```python
from build123d import *

# Parameters (mm, degrees)
PAD_DEPTH       = 7
PAD012_DEPTH    = 25
SKETCH013_R     = 5
SKETCH013_R_2   = 3
POCKET007_DEPTH = 7.001
POCKET008_DEPTH = 30
SKETCH023_R     = 5
POCKET009_DEPTH = 4
SKETCH024_R     = 4.5
PAD013_DEPTH    = 30
SKETCH028_R     = 2.75
POCKET012_DEPTH = 1.5
SKETCH029_R     = 1.55
POCKET013_DEPTH = 32.001
SKETCH030_R     = 2.5
POCKET014_DEPTH = 3
POCKET015_DEPTH = 25.001


with BuildPart() as part:
    # Sketch011 → Pad (new body)
    with BuildSketch(Plane.XZ):
        with BuildLine():
            Line((73.255, 35.51), (73.255, 5))
            ThreePointArc((68.255, 0), (71.790534, 1.464466), (73.255, 5))
            Line((68.255, 0), (-68.255, 0))
            ThreePointArc((-73.255, 5), (-71.790534, 1.464466), (-68.255, 0))
            Line((-73.255, 5), (-73.255, 35.51))
            Line((-73.255, 35.51), (-81.66, 35.51))
            ThreePointArc((-86.66, 40.51), (-85.195534, 36.974466), (-81.66, 35.51))
            Line((-86.66, 40.51), (-86.66, 79.371844))
            ThreePointArc((-79.132903, 89.061258), (-84.557121, 85.50662), (-86.66, 79.371844))
            ThreePointArc((79.132903, 89.061258), (0, 99), (-79.132903, 89.061258))
            ThreePointArc((86.66, 79.371844), (84.557121, 85.50662), (79.132903, 89.061258))
            Line((86.66, 79.371844), (86.66, 40.51))
            ThreePointArc((81.66, 35.51), (85.195534, 36.974466), (86.66, 40.51))
            Line((81.66, 35.51), (73.255, 35.51))
        make_face()
    extrude(amount=PAD_DEPTH)

    # Sketch012 → Pad012 (join)
    with BuildSketch(Plane.XZ):
        with BuildLine():
            ThreePointArc((79.132903, 89.061258), (0, 99), (-79.132903, 89.061258))
            ThreePointArc((-79.132903, 89.061258), (-84.557121, 85.50662), (-86.66, 79.371844))
            Line((-86.66, 79.371844), (-86.66, 40.51))
            ThreePointArc((-86.66, 40.51), (-85.195534, 36.974466), (-81.66, 35.51))
            Line((-81.66, 35.51), (-73.255, 35.51))
            Line((-73.255, 35.51), (-73.255, 28.649016))
            ThreePointArc((-73.255, 28.649016), (-53.725584, 32.7828), (-34.688969, 38.790593))
            ThreePointArc((34.688969, 38.790593), (0, 45), (-34.688969, 38.790593))
            ThreePointArc((34.688969, 38.790593), (53.725584, 32.7828), (73.255, 28.649016))
            Line((73.255, 35.51), (73.255, 28.649016))
            Line((73.255, 35.51), (81.66, 35.51))
            ThreePointArc((81.66, 35.51), (85.195534, 36.974466), (86.66, 40.51))
            Line((86.66, 40.51), (86.66, 79.371844))
            ThreePointArc((86.66, 79.371844), (84.557121, 85.50662), (79.132903, 89.061258))
        make_face()
    extrude(amount=-PAD012_DEPTH)

    # Sketch013 → Pocket007 (cut, through all)
    with BuildSketch(Plane.XZ):
        with Locations((-50, 14)):
            Circle(SKETCH013_R)
        with Locations((-28, 14)):
            Circle(SKETCH013_R_2)
        with Locations((28, 14)):
            Circle(SKETCH013_R_2)
        with Locations((50, 14)):
            Circle(SKETCH013_R)
    extrude(amount=POCKET007_DEPTH, mode=Mode.SUBTRACT)

    # Sketch015 → Pocket008 (cut)
    with BuildSketch(Plane.XZ.offset(7)):
        with BuildLine():
            Line((81.66, 75.603787), (81.66, 45.51))
            ThreePointArc((76.66, 40.51), (80.195534, 41.974466), (81.66, 45.51))
            Line((76.66, 40.51), (68.255, 40.51))
            Line((68.255, 40.51), (68.255, 34.519539))
            ThreePointArc((34.688969, 43.790593), (51.275394, 38.443308), (68.255, 34.519539))
            ThreePointArc((34.688969, 43.790593), (0, 50), (-34.688969, 43.790593))
            ThreePointArc((-68.255, 34.519539), (-51.275394, 38.443308), (-34.688969, 43.790593))
            Line((-68.255, 40.51), (-68.255, 34.519539))
            Line((-76.66, 40.51), (-68.255, 40.51))
            ThreePointArc((-81.66, 45.51), (-80.195534, 41.974466), (-76.66, 40.51))
            Line((-81.66, 45.51), (-81.66, 75.603787))
            ThreePointArc((-73.971613, 85.332942), (-79.505895, 81.803943), (-81.66, 75.603787))
            ThreePointArc((73.971613, 85.332942), (0, 94), (-73.971613, 85.332942))
            ThreePointArc((81.66, 75.603787), (79.505895, 81.803943), (73.971613, 85.332942))
        make_face()
    extrude(amount=-POCKET008_DEPTH, mode=Mode.SUBTRACT)

    # Sketch023 → Pocket009 (cut)
    with BuildSketch(Plane.XZ.offset(7)):
        with Locations((-28, 14)):
            Circle(SKETCH023_R)
        with Locations((28, 14)):
            Circle(SKETCH023_R)
    extrude(amount=-POCKET009_DEPTH, mode=Mode.SUBTRACT)

    # Sketch024 → Pad013 (join)
    with BuildSketch(Plane.XZ.offset(-23)):
        with Locations((-79.61305, 81.665882)):
            Circle(SKETCH024_R)
        with Locations((79.61305, 81.665882)):
            Circle(SKETCH024_R)
    extrude(amount=PAD013_DEPTH)

    # Sketch028 → Pocket012 (cut)
    with BuildSketch(Plane.XZ.offset(7)):
        with Locations((-66.789089, 6.465911)):
            Circle(SKETCH028_R)
        with Locations((66.789089, 6.465911)):
            Circle(SKETCH028_R)
    extrude(amount=-POCKET012_DEPTH, mode=Mode.SUBTRACT)

    # Sketch029 → Pocket013 (cut, through all)
    with BuildSketch(Plane.XZ.offset(-25)):
        with Locations((-79.61305, 81.665882)):
            Circle(SKETCH029_R)
        with Locations((79.61305, 81.665882)):
            Circle(SKETCH029_R)
    extrude(amount=POCKET013_DEPTH, mode=Mode.SUBTRACT)

    # Sketch030 → Pocket014 (cut)
    with BuildSketch(Plane.XZ.offset(-25)):
        with Locations((-79.61305, 81.665882)):
            Circle(SKETCH030_R)
        with Locations((79.61305, 81.665882)):
            Circle(SKETCH030_R)
    extrude(amount=POCKET014_DEPTH, mode=Mode.SUBTRACT)

    # Sketch031 → Pocket015 (cut, through all)
    with BuildSketch(Plane.XZ):
        with BuildLine():
            ThreePointArc((53.201861, 82.094664), (49.201861, 78.094664), (53.201861, 74.094664))
            Line((53.201861, 74.094664), (63.201861, 74.094664))
            ThreePointArc((63.201861, 74.094664), (67.201861, 78.094664), (63.201861, 82.094664))
            Line((63.201861, 82.094664), (53.201861, 82.094664))
        make_face()
    extrude(amount=-POCKET015_DEPTH, mode=Mode.SUBTRACT)


solid = part.part
```
The model under review builds one solid part; all positions refer to its coordinate system, in mm. A direction names the side the tool comes from. Round coordinates to 2 decimals unless told otherwise and drop trailing zeros. Write each loop counter-clockwise with the first axis right and the second up, starting at its lowest first coordinate (ties: lowest second). Pieces come first, ordered by that corner, then holes.
(1) Wall thickness on L1, parallel to X at y = 7.5, z = 53; L2, parallel to X at y = -2.5, z = 13 (3 decimals); L3, parallel to Z at x = -50, y = -2.5: over which ranges is each line inside the solid? List them lowest first.
(2) We need section C-C on y = 2.5. Give the number of separate pieces and of enclosed holes in the cut face, and give its area (3 significant figures).
(3) Machinability: for faces 1 (the cylindrical face through (-80.23, 7.79, 42.01)), 2 (the cylindrical face through (77.77, 23.521, 83.356)), 3 (the cylindrical face through (-54, 12.32, 32.71)), 4 (the cylindrical face through (-84.5, 8.78, 85.58)), 5 (the cylindrical face through (-78.135, 7.703, 82.131)), which of the approach directions +Z, -Z, +X, -X, +Y, -Y give a long, thin tool a straight path to every point of the face, cutting with its end or side? Answer none if there is none.
(4) We need section B-B on z = 56. Give the boundary of the cut face in (x, y), and give its area (3 significant figures).
(5) We need section A-A on x = 28. Give the boundary of the cut face in (y, z), and give its area (3 significant figures).
(6) Insertion check: pin 1 (10 mm diameter, centred on x = -9, y = 7.5, fed in from -Z); pin 2 (8 mm diameter, centred on x = 56, z = 10, fed in from +Y); pin 3 (9 mm diameter, centred on x = 28, z = 14, fed in from -Y). Each pin has a flat end and moves straight along its axis. Give the tip position at first contact, or say it passes through.
(7) Mouldability with a two-part tool opening along X and no side actions: class faces 6 (the flat face through (-80, 22, 80)), 7 (the flat face through (1, 0, 18)), 8 (the cylindrical face through (-71.829, -3.451, 1.504)), 9 (the flat face through (-1, -7, 39)) as +X half, -X half, draft (parallel to the pull), parting line (faces both ways), or undercut.
(8) We need section D-D on x = -50. Give the boundary of the cut face in (y, z).
Findings below:
1. L1: x = -86.66 to -81.66, 81.66 to 86.66
1. L2: x = -73.255 to -54.899, -45.101 to -30.828, -25.172 to 25.172, 30.828 to 45.101, 54.899 to 73.255
1. L3: z = 0 to 9, 19 to 38.8, 90.07 to 95.07
2. separate pieces: 1
2. enclosed holes: 3
2. area: 2,260 mm2
3. face 1: -Y
3. face 2: +Y
3. face 3: -Z, +Y
3. face 4: +Z, -X, +Y, -Y
3. face 5: +Y, -Y
4. outline: (-86.66, -7) - (-81.66, -7) - (-81.66, 23) - (81.66, 23) - (81.66, -7) - (86.66, -7) - (86.66, 25) - (-86.66, 25) - close
4. area: 647 mm2
5. outline: (-7, 0) - (0, 0) - (0, 11) - (-3, 11) - (-3, 9) - (-7, 9) - close; (-7, 19) - (-3, 19) - (-3, 17) - (0, 17) - (0, 41) - (25, 41) - (25, 97.77) - (-7, 97.77) - (-7, 92.77) - (23, 92.77) - (23, 46) - (-7, 46) - close
5. area: 643 mm2
6. pin 1: stops at z = 44.02
6. pin 2: stops at y = 0
6. pin 3: stops at y = -3
7. face 6: undercut
7. face 7: undercut
7. face 8: -X half
7. face 9: draft
8. outline: (-7, 0) - (0, 0) - (0, 9) - (-7, 9) - close; (-7, 19) - (0, 19) - (0, 33.8) - (25, 33.8) - (25, 95.07) - (-7, 95.07) - (-7, 90.07) - (23, 90.07) - (23, 38.8) - (-7, 38.8) - close
